```python
from build123d import *

# Parameters (mm, degrees)
SKETCH1_R           = 1.75
BOSS_EXTRUDE1_DEPTH = 1.6
SKETCH2_W           = 5.933953942
SKETCH2_H           = 8.053817615
SKETCH2_W_2         = 3.324070188
SKETCH2_H_2         = 4.276777171
SKETCH2_W_3         = 2.922259506
SKETCH2_H_3         = 1.680299216
BOSS_EXTRUDE2_DEPTH = 3.1
SKETCH3_W           = 3.740844247
SKETCH3_H           = 4.973122352
SKETCH3_W_2         = 11.134512877
SKETCH3_H_2         = 14.391247869
BOSS_EXTRUDE3_DEPTH = 3.1
SKETCH4_W           = 6.597488945
SKETCH4_H           = 2.482560273
CUT_EXTRUDE1_DEPTH  = 5.1


with BuildPart() as part:
    # Sketch1 → Boss-Extrude1 (new body)
    with BuildSketch(Plane(origin=(0, 0, 0), x_dir=(1, 0, 0), z_dir=(0, 1, 0))):
        with BuildLine():
            Line((-8.692785485, -16), (8.692785485, -16))
            add(Edge.make_bspline(
                [(15, -9.18383354), (14.366330033, -12.951143486), (10.86731964, -13.80158376), (8.692785485, -16)],
                knots=[0, 0, 0, 0, 0.915310456, 0.915310456, 0.915310456, 0.915310456], degree=3))
            Line((15, -9.18383354), (15, 12.5))
            ThreePointArc((15, 12.5), (13.974873734, 14.974873734), (11.5, 16))
            Line((11.5, 16), (8.692785485, 16))
            Line((8.692785485, 16), (8.692785485, 15.700659593))
            ThreePointArc((8.692785485, 15.700659593), (8.546338876, 15.347106203), (8.192785485, 15.200659593))
            Line((8.192785485, 15.200659593), (-8.192785485, 15.200659593))
            ThreePointArc((-8.192785485, 15.200659593), (-8.546338876, 15.347106203), (-8.692785485, 15.700659593))
            Line((-8.692785485, 15.700659593), (-8.692785485, 16))
            Line((-8.692785485, 16), (-11.5, 16))
            ThreePointArc((-11.5, 16), (-13.974873734, 14.974873734), (-15, 12.5))
            Line((-15, 12.5), (-15, -9.18383354))
            add(Edge.make_bspline(
                [(-15, -9.18383354), (-14.366330033, -12.951143486), (-10.86731964, -13.80158376), (-8.692785485, -16)],
                knots=[0, 0, 0, 0, 0.915310456, 0.915310456, 0.915310456, 0.915310456], degree=3))
        make_face()
        with Locations(Location((-10, 10, 0), (0, 0, 270))):
            Circle(SKETCH1_R, mode=Mode.SUBTRACT)
        with Locations(Location((10, 10, 0), (0, 0, 270))):
            Circle(SKETCH1_R, mode=Mode.SUBTRACT)
        with Locations(Location((10, -10, 0), (0, 0, 270))):
            Circle(SKETCH1_R, mode=Mode.SUBTRACT)
        with Locations(Location((-10, -10, 0), (0, 0, 270))):
            Circle(SKETCH1_R, mode=Mode.SUBTRACT)
    extrude(amount=BOSS_EXTRUDE1_DEPTH)

    # Sketch2 → Boss-Extrude2 (add)
    with BuildSketch(Plane(origin=(0, 1.6, 0), x_dir=(1, 0, 0), z_dir=(0, 1, 0))):
        with Locations((12.033023029, 0.352079458)):
            Rectangle(SKETCH2_W, SKETCH2_H)
        with Locations((-7.946367365, 3.796471816)):
            Rectangle(SKETCH2_W_2, SKETCH2_H_2)
        with Locations((-4.311807104, -5.315838698)):
            Rectangle(SKETCH2_W_3, SKETCH2_H_3)
    extrude(amount=BOSS_EXTRUDE2_DEPTH)

    # Sketch3 → Boss-Extrude3 (add)
    with BuildSketch(Plane.XZ):
        with Locations((-10.100279468, -2.904655533)):
            Rectangle(SKETCH3_W, SKETCH3_H)
        with Locations((0.902203613, 0.616139053)):
            Rectangle(SKETCH3_W_2, SKETCH3_H_2)
    extrude(amount=BOSS_EXTRUDE3_DEPTH)

    # Sketch4 → Cut-Extrude1 (cut)
    with BuildSketch(Plane(origin=(15, 0, 0), x_dir=(0, 0, -1), z_dir=(1, 0, 0))):
        with Locations((0.34007675, 2.942483523)):
            Rectangle(SKETCH4_W, SKETCH4_H)
    extrude(amount=-CUT_EXTRUDE1_DEPTH, mode=Mode.SUBTRACT)


solid = part.part
```
Here's how the part is built. I have some questions about the finished solid (model axes, mm). A direction names the side the tool comes from. Coordinates: 2 decimals unless noted, no trailing zeros. Loops run counter-clockwise (first coordinate to the right, second up) from the corner with the lowest first, then second, coordinate; pieces in that order, holes last. Notation, with made-up numbers: M 27,40 L 36,40 A19 cw 36,52 Z; hole C 2.25,31 d5. An arc over 180 degrees is marked long. One line per item, written item: value.
1. Imagine slicing it at A-A (y = -1). List the corners of the cut face in (x, z) for me.
Geometry says:
outline: M -11.97,-5.39 L -8.23,-5.39 L -8.23,-0.42 L -11.97,-0.42 Z; M -4.67,-6.58 L 6.47,-6.58 L 6.47,7.81 L -4.67,7.81 Z
2. On a 3-axis mill with a long thin cutter (end or side, diameter ignored), from which of +Z, -Z, +X, -X, +Y, -Y can I reach the whole of each face in a straight line? I mean faces 4 (the flat face through (9.066, 3, 0)), 5 (the flat face through (-11.971, -2, -3)), 6 (the flat face through (12, 3, -3.639)), 7 (the flat face through (-4.665, -2, 1)). Say none if no direction works.
Geometry says:
face 4: +Z, -Z, +Y
face 5: +Z, -Z, -X, -Y
face 6: +X
face 7: +Z, -Z, -Y
3. Imagine slicing it at B-B (z = -10). List the corners of the cut face in (x, y) for me, and give its area (3 significant figures).
Geometry says:
outline: M -15,0 L -11.75,0 L -11.75,1.6 L -15,1.6 Z; M -8.25,0 L 8.25,0 L 8.25,1.6 L -8.25,1.6 Z; M 11.75,0 L 15,0 L 15,1.6 L 11.75,1.6 Z
area: 36.8 mm2
4. Please list where these lines run through material, in increasing order: probe 1 along Z at (x, y) = (-11, 0.75); probe 2 along X at (y, z) = (0.5, 11); probe 3 along X at (y, z) = (0.85, 10).
Geometry says:
probe 1: z = -16 to -11.44, -8.56 to 8.56, 11.44 to 14.2
probe 2: x = -14.38 to -11.44, -8.56 to 8.56, 11.44 to 14.38
probe 3: x = -14.81 to -11.75, -8.25 to 8.25, 11.75 to 14.81
5. Imagine slicing it at D-D (x = -7). List the corners of the cut face in (y, z) for me.
Geometry says:
outline: M 0,-15.2 L 1.6,-15.2 L 1.6,-5.93 L 4.7,-5.93 L 4.7,-1.66 L 1.6,-1.66 L 1.6,16 L 0,16 Z
6. Thinking about a two-plate mould opening in Y: for faces 1 (the cylindrical face through (14, 0.79, -14.95)), 2 (the flat face through (-10, -3.1, -3)), 3 (the flat face through (12, 4.184, 0)), which applies, +Y half, -Y half, draft (parallel to the pull), parting line (faces both ways), or undercut?
Geometry says:
face 1: draft
face 2: -Y half
face 3: undercut
7. Will these pins go through, and if not, where does the flat tip stop? pin 1 Ø0.9 at (y, z) = (4, -3.5) entering from +X; pin 2 Ø1.6 at (x, y) = (10.5, 3.5) entering from +Z; pin 3 Ø1.6 at (x, y) = (-10, -2) entering from -Z; pin 4 Ø3.5 at (y, z) = (-2, -4) entering from -X.
Geometry says:
pin 1: stops at x = 15
pin 2: stops at z = 3.67
pin 3: stops at z = -5.39
pin 4: stops at x = -11.97
8. Imagine slicing it at C-C (y = 2.75). List the corners of the cut face in (x, z) for me.
Geometry says:
outline: M -9.61,-5.93 L -6.28,-5.93 L -6.28,-1.66 L -9.61,-1.66 Z; M -5.77,4.48 L -2.85,4.48 L -2.85,6.16 L -5.77,6.16 Z; M 9.07,-4.38 L 15,-4.38 L 15,-3.64 L 9.9,-3.64 L 9.9,2.96 L 15,2.96 L 15,3.67 L 9.07,3.67 Z
